CAD build for the part. Positions are in the model's coordinates, mm. A direction names the side the tool comes from. Round coordinates to 2 decimals unless told otherwise and drop trailing zeros. Write each loop counter-clockwise with the first axis right and the second up, starting at its lowest first coordinate (ties: lowest second). Pieces come first, ordered by that corner, then holes. Notation, with made-up numbers: (53.5, 51) - (71.5, 51) arc R21 cw to (71.5, 58) - close; hole circle Ø11 at (77, -39). An arc over 180 degrees is marked (long way). Put each result on its own line as item: value. Start each with the question number.
Item 1: Cut at B-B (z = -0.5). Give the cut face in (x, y).
Item 2: 3-axis set-ups, long thin cutter, end or side, ignore diameter. For faces 1 (the flat face through (122, -25.409, 0)), 2 (the flat face through (122, -19.059, 0)): which of +Z, -Z, +X, -X, +Y, -Y reach the whole face in a straight line?
Item 3: Cut at D-D (y = 21.5). Give the cut face in (x, z).
Item 4: Cut at C-C (y = 0). Give the cut face in (x, z), and give its area (3 significant figures).
Item 5: Pin check, flat tips, straight feed: pin 1 Ø1 at (y, z) = (-5.5, -0.5) entering from +X; pin 2 Ø3 at (y, z) = (-2.5, 2) entering from +X. Stop position of each tip, or through.
Item 6: Mould opens along Z. For faces 3 (the cylindrical face through (266.704, 0.419, -0.053)), 4 (the flat face through (123, 21, -3.81)), 5 (the flat face through (123, 21, 3.81)) say: released by +Z, released by -Z, zero draft, split by the parting line, or undercut.
Item 7: Drill centre lines: line 1 (Y direction, x = 206, z = 3); line 2 (X direction, y = 1, z = -3); line 3 (X direction, y = 1.5, z = -1). Where is each one in solid material? Low to high. Write a range as from..to.
Item 8: Cut at A-A (x = 216.5). Give the cut face in (y, z).
Autodesk Inventor part; units mm, degrees
ref_plane "YZ Plane" through (0, 0, 0) normal (1, 0, 0) x (0, 1, 0)
ref_plane "XZ Plane" through (0, 0, 0) normal (0, 1, 0) x (-1, 0, 0)
ref_plane "XY Plane" through (0, 0, 0) normal (0, 0, 1) x (1, 0, 0)
sketch "Sketch1" plane through (0, 0, 0) normal (0, 0, 1) x (1, 0, 0)
  line L0 (0, 22.2339) -> (247.65, 22.2339) construction
  line L1 (0, -22.2339) -> (247.65, -22.2339) construction
  arc A0 (0, 22.2339) -> (0, -22.2339) centre (0, 0) ccw construction
  line L2 (0, 0) -> (247.65, 0) construction
  arc A1 (247.65, -22.2339) -> (247.65, 22.2339) centre (247.65, 0) ccw construction
  line L3 (247.65, 25.4089) -> (0, 25.4089)
  arc A2 (0, 25.4089) -> (0, -25.4089) centre (0, 0) ccw
  line L4 (0, -25.4089) -> (247.65, -25.4089)
  arc A3 (247.65, -25.4089) -> (247.65, 25.4089) centre (247.65, 0) ccw
  line L5 (247.65, 19.0589) -> (0, 19.0589)
  arc A4 (0, 19.0589) -> (0, -19.0589) centre (0, 0) ccw
  line L6 (0, -19.0589) -> (247.65, -19.0589)
  arc A5 (247.65, -19.0589) -> (247.65, 19.0589) centre (247.65, 0) ccw
  dimension "d1" = 22.234
  dimension "d2" = 22.234
  dimension "d3" = 3.175
  dimension "d4" = 3.175
  dimension "CtoC" = 247.65
extrude "Extrusion1" add sketch "Sketch1" along normal mid plane 7.62
properties part number "25 Chain Template" material "Silicon Nitride"
Output values:
1. outline: (0, -25.41) - (247.65, -25.41) arc R25.41 ccw to (247.65, 25.41) - (0, 25.41) arc R25.41 ccw to start; hole (0, -19.06) - (247.65, -19.06) arc R19.06 ccw to (247.65, 19.06) - (0, 19.06) arc R19.06 ccw to start
2. face 1: +Z, -Z, +X, -X, -Y
2. face 2: +Z, -Z
3. outline: (-13.54, -3.81) - (261.19, -3.81) - (261.19, 3.81) - (-13.54, 3.81) - close
4. outline: (-25.41, -3.81) - (-19.06, -3.81) - (-19.06, 3.81) - (-25.41, 3.81) - close; (266.71, -3.81) - (273.06, -3.81) - (273.06, 3.81) - (266.71, 3.81) - close
4. area: 96.8 mm2
5. pin 1: x = 272.56
5. pin 2: x = 273.04
6. face 3: zero draft
6. face 4: released by -Z
6. face 5: released by +Z
7. line 1: -25.41..-19.06, 19.06..25.41
7. line 2: -25.39..-19.03, 266.68..273.04
7. line 3: -25.36..-19, 266.65..273.01
8. outline: (-25.41, -3.81) - (-19.06, -3.81) - (-19.06, 3.81) - (-25.41, 3.81) - close; (19.06, -3.81) - (25.41, -3.81) - (25.41, 3.81) - (19.06, 3.81) - close
